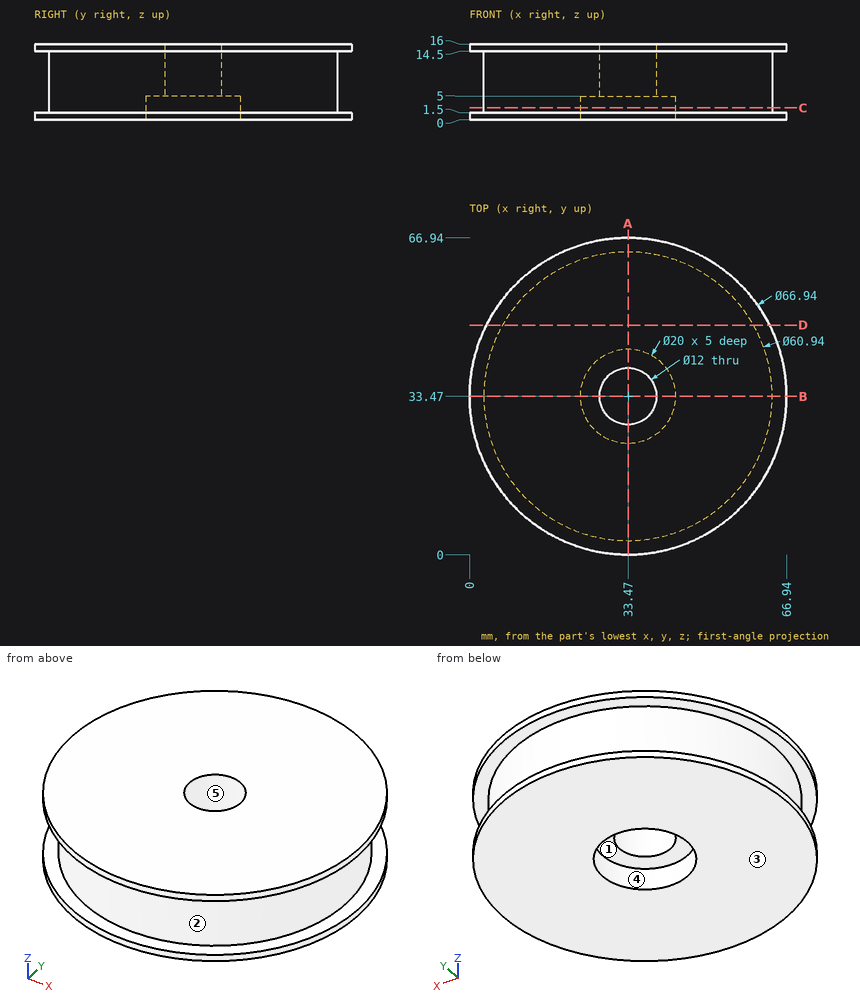
The drawing under review shows one solid part. Ordinate dimensions are in mm from its lowest x, y, z. A direction names the side the tool comes from. Round coordinates to 2 decimals unless told otherwise and drop trailing zeros. Write each loop counter-clockwise with the first axis right and the second up, starting at its lowest first coordinate (ties: lowest second). Pieces come first, ordered by that corner, then holes. Notation, with made-up numbers: (-38, 35.5) - (-2, 35.5) arc R32 cw to (-2, 70.5) - close; hole circle Ø7 at (28, 38.25). An arc over 180 degrees is marked (long way). One line per question, with ' | ' between items.
Item 1: To check wall thickness, follow probe 1 along Y at (x, z) = (33.47, 8.75); probe 2 along Y at (x, z) = (33.47, 3.15); probe 3 along Z at (x, y) = (4, 41.5). State the ranges of each line that lie inside material, in increasing order.
Resolved:
probe 1: y = 3 to 27.47, 39.47 to 63.94 | probe 2: y = 3 to 23.47, 43.47 to 63.94 | probe 3: z = 0 to 1.5, 14.5 to 16
Item 2: Add section D-D, the plane y = 48.5. Give the boundary of the cut face in (x, z), then the cut area to 3 significant figures.
Resolved:
outline: (3.56, 0) - (63.38, 0) - (63.38, 1.5) - (59.98, 1.5) - (59.98, 14.5) - (63.38, 14.5) - (63.38, 16) - (3.56, 16) - (3.56, 14.5) - (6.96, 14.5) - (6.96, 1.5) - (3.56, 1.5) - close | area: 869 mm2
Item 3: For P1, Ø6, axis at y = 18.5, z = 5.5, coming from the +X side; P2, Ø9.5, axis at x = 33.47, y = 33.47, coming from the +Z side; P3, Ø1.5, axis at x = 31, y = 39, coming from the -Z side; P4, Ø8, axis at x = 26.5, y = 55, coming from the -Z side, all flat-tipped, find the tip position at first contact; note any pin that passes through.
Resolved:
P1: stops at x = 61.49 | P2: passes through | P3: stops at z = 5 | P4: stops at z = 0
Item 4: The part is to be moulded in two halves that separate along X. For the marked faces 1, 2 and 3, say which applies: pulls with the +X half, pulls with the -X half, needs draft (parallel to the pull), parting line crosses it, or undercut.
Resolved:
face 1: undercut | face 2: parting line crosses it | face 3: needs draft
Item 5: For the marked faces 4 and 5, list the 3-axis set-ups (+Z, -Z, +X, -X, +Y, -Y) from which the entire face can be reached by the end or side of a thin tool; tool diameter is ignored.
Resolved:
face 4: -Z | face 5: +Z, -Z
Item 6: Add section A-A, the plane x = 33.47. Give the boundary of the cut face in (y, z).
Resolved:
outline: (0, 0) - (23.47, 0) - (23.47, 5) - (27.47, 5) - (27.47, 16) - (0, 16) - (0, 14.5) - (3, 14.5) - (3, 1.5) - (0, 1.5) - close; (39.47, 5) - (43.47, 5) - (43.47, 0) - (66.94, 0) - (66.94, 1.5) - (63.94, 1.5) - (63.94, 14.5) - (66.94, 14.5) - (66.94, 16) - (39.47, 16) - close
Item 7: Add section C-C, the plane z = 2.5. Give the boundary of the cut face in (x, y).
Resolved:
outline: circle Ø60.94 at (33.47, 33.47); hole circle Ø20 at (33.47, 33.47)
